Verification items for the finished model (mm, model axes). A direction names the side the tool comes from. Coordinates: 2 decimals unless noted, no trailing zeros. Order: outer loops, then holes, each group sorted by start corner. A loop starts at its lowest first (then second) coordinate and runs counter-clockwise, first axis right, second up. Notation, with made-up numbers: (73, -27) -> (115, -27) arc R14 ccw to (115, -15) -> close; hole circle Ø10 at (-18, -6.75). An arc over 180 degrees is marked (long way). Use CSV: the item, a comma, the result in double quotes. Start each with the question number.
1) Go/stop test with flat-tipped pins: pin 1 (1 mm diameter, centred on y = 0, z = -20.5, fed in from +X); pin 2 (4 mm diameter, centred on y = -1.5, z = -9.5, fed in from +X); pin 3 (1.5 mm diameter, centred on x = -3.5, y = 4.5, fed in from +Z); pin 4 (2.5 mm diameter, centred on x = -0.5, z = -10.5, fed in from +Y). Record where each tip stops, or that it passes through.
2) Sectioned sample at C-C on z = -18. Record the boundary of the cut face in (x, y).
3) Sectioned sample at D-D on z = -4.5. Record the boundary of the cut face in (x, y).
4) Tool access check on faces 4 (the cylindrical face through (3.97, 0.05, -10.81)), 5 (the flat face through (0.127, 0, -20)), 6 (the cylindrical face through (-0.27, 2.09, -7.96)), 7 (the flat face through (0, -2.972, -11)). Record the directions out of +Z, -Z, +X, -X, +Y, -Y that give a thin tool (end or side, any length) a straight path to the whole face; none if there is none.
5) Sectioned sample at A-A on y = 0. Record the boundary of the cut face in (x, z) (3 decimals).
6) Release check for a two-part mould opening along Y. For faces 1 (the flat face through (0, 0, -15.875)), 2 (the cylindrical face through (-3.97, -0.05, -10.81)), 3 (the flat face through (0, 4, -4.775)) record: released by +Y, released by -Y, zero draft, split by the parting line, or undercut.
7) Scan lines: line 1 along Y through (x, z) = (0, -4); line 2 along Y through (x, z) = (0, -10); line 3 along Z through (x, y) = (-3, 1.75). Record each from-to range of solid material in increasing order.
8) Sectioned sample at B-B on z = -7. Record the boundary of the cut face in (x, y).
from build123d import *

# Parameters (mm, degrees)
FILLET1_R           = 0.508
SKETCH2_OUTSIDE_W   = 17.714
SKETCH2_OUTSIDE_H   = 17.714
SKETCH2_OUTSIDE_W_2 = 9.40445076
SKETCH2_OUTSIDE_H_2 = 5.9436
CUT_EXTRUDE1_DEPTH  = 11.9126
SKETCH3_W           = 0.254
SKETCH3_H           = 3.175
BOSS_EXTRUDE1_DEPTH = 7.1374
SKETCH4_R           = 1.1938
CUT_EXTRUDE2_DEPTH  = 7.1374
CUT_EXTRUDE3_DEPTH  = 7.1374
SKETCH7_R           = 2.1082
CUT_EXTRUDE4_DEPTH  = 15.875
CHAMFER2_SIZE       = 0.254


with BuildPart() as part:
    # Sketch1 → Revolve1 (revolve)
    with BuildSketch(Plane(origin=(0, 0, 0), x_dir=(0, 0, -1), z_dir=(1, 0, 0)), mode=Mode.PRIVATE) as revolve1_sk:
        Polygon((0, 0), (0, 5.5626), (4.7752, 5.5626), (4.7752, 3.96875), (16.6878, 3.96875), (16.6878, 0), align=None)
    revolve(revolve1_sk.sketch.rotate(Axis((0, 0, 0), (0, 0, -1)), 90), axis=Axis((0, 0, 0), (0, 0, -1)))  # turned: the seam where the file's is

    # Fillet1
    fillet1_edges = [part.edges().sort_by_distance(p)[0] for p in [
        (-5.5626, 0, 0),
    ]]
    fillet(fillet1_edges, radius=FILLET1_R)

    # Sketch2 outside → Cut-Extrude1 (cut)
    with BuildSketch(Plane(origin=(0, 0, -16.6878), x_dir=(-1, 0, 0), z_dir=(0, 0, -1))):
        Rectangle(SKETCH2_OUTSIDE_W, SKETCH2_OUTSIDE_H)
        Rectangle(SKETCH2_OUTSIDE_W_2, SKETCH2_OUTSIDE_H_2, mode=Mode.SUBTRACT)
    extrude(amount=-CUT_EXTRUDE1_DEPTH, mode=Mode.SUBTRACT)

    # Sketch3 → Boss-Extrude1 (add)
    with BuildSketch(Plane(origin=(0, 0, -16.6878), x_dir=(-1, 0, 0), z_dir=(0, 0, -1))):
        Rectangle(SKETCH3_W, SKETCH3_H)
    extrude(amount=BOSS_EXTRUDE1_DEPTH)

    # Sketch4 → Cut-Extrude2 (cut)
    with BuildSketch(Plane.ZY.offset(0.127)):
        with Locations((-21.9202, 0)):
            Circle(SKETCH4_R)
    extrude(amount=-CUT_EXTRUDE2_DEPTH, mode=Mode.SUBTRACT)

    # Sketch5 → Cut-Extrude3 (cut)
    with BuildSketch(Plane.ZY.offset(0.127)):
        Polygon((-16.6878, 1.5875), (-16.6878, 1.2065), (-17.3228, 1.5875), align=None)
        Polygon((-16.6878, -1.2065), (-17.3228, -1.5875), (-16.6878, -1.5875), align=None)
    extrude(amount=-CUT_EXTRUDE3_DEPTH, mode=Mode.SUBTRACT)

    # Sketch7 → Cut-Extrude4 (cut)
    with BuildSketch(Plane.XY):
        Circle(SKETCH7_R)
    extrude(amount=-CUT_EXTRUDE4_DEPTH, mode=Mode.SUBTRACT)

    # Chamfer2
    chamfer2_edges = [part.edges().sort_by_distance(p)[0] for p in [
        (-2.1082, 0, 0),
    ]]
    chamfer(chamfer2_edges, length=CHAMFER2_SIZE)


solid = part.part
Answers follow:
1,pin 1,"stops at x = 0.13"
1,pin 2,"stops at x = 3.97"
1,pin 3,"stops at z = 0"
1,pin 4,"stops at y = 2.97"
2,outline,"(-0.13, -1.59) -> (0.13, -1.59) -> (0.13, 1.59) -> (-0.13, 1.59) -> close"
3,outline,"circle Ø11.13 at (0, 0); hole circle Ø4.22 at (0, 0)"
4,face 4,"-Z, +X"
4,face 5,"-Z, +X, +Y, -Y"
4,face 6,"+Z"
4,face 7,"-Z, +X, -X, -Y"
5,outline,"(-5.563, -4.775) -> (-3.969, -4.775) -> (-3.969, -16.688) -> (-0.127, -16.688) -> (-0.127, -20.726) -> (0.127, -20.726) -> (0.127, -16.688) -> (3.969, -16.688) -> (3.969, -4.775) -> (5.563, -4.775) -> (5.563, -0.508) arc R0.508 ccw to (5.055, 0) -> (2.362, 0) -> (2.108, -0.254) -> (2.108, -15.875) -> (-2.108, -15.875) -> (-2.108, -0.254) -> (-2.362, 0) -> (-5.055, 0) arc R0.508 ccw to (-5.563, -0.508) -> close; (-0.127, -23.825) -> (0.127, -23.825) -> (0.127, -23.114) -> (-0.127, -23.114) -> close"
6,face 1,"undercut"
6,face 2,"split by the parting line"
6,face 3,"zero draft"
7,line 1,"y = -5.56 to -2.11, 2.11 to 5.56"
7,line 2,"y = -2.97 to -2.11, 2.11 to 2.97"
7,line 3,"z = -16.69 to 0"
8,outline,"(-2.63, -2.97) -> (2.63, -2.97) arc R3.97 ccw to (2.63, 2.97) -> (-2.63, 2.97) arc R3.97 ccw to start; hole circle Ø4.22 at (0, 0)"
